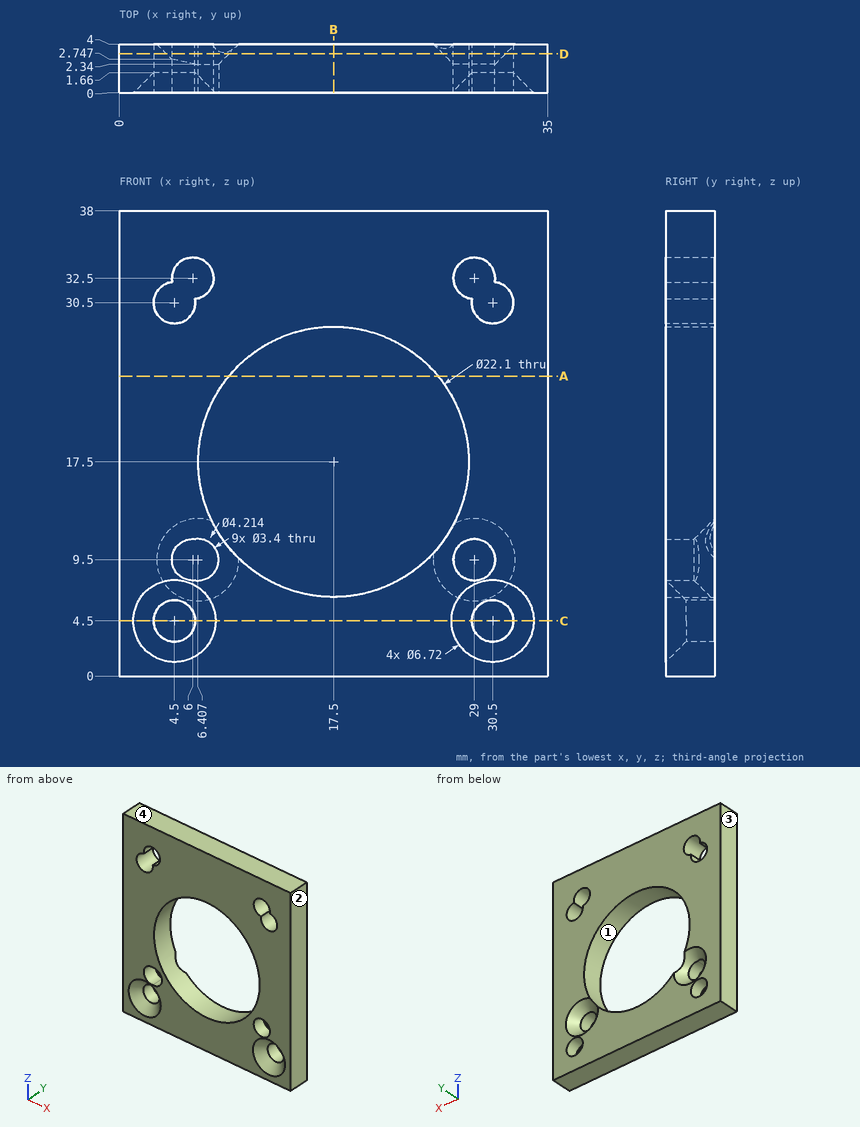
The drawing under review shows one solid part. Ordinate dimensions are in mm from its lowest x, y, z. Coordinates: 2 decimals unless noted, no trailing zeros. Order: outer loops, then holes, each group sorted by start corner. A loop starts at its lowest first (then second) coordinate and runs counter-clockwise, first axis right, second up. Notation, with made-up numbers: (-11.75, -26) -> (32.25, -26) arc R21 cw to (32.25, -13) -> close; hole circle Ø2 at (17, 13.25). An arc over 180 degrees is marked (long way). Answer in a Markdown table with one row per item. Add a question column.
Item 1: Clearance check with flat-ended pins moving along their axes: pin 1 (2 mm diameter, centred on x = 6, z = 32.5, fed in from +Y); pin 2 (5.5 mm diameter, centred on x = 4.5, z = 4.5, fed in from -Y); pin 3 (5.5 mm diameter, centred on x = 6.41, z = 9.5, fed in from +Y). State where each tip first meets the part, or that it passes through.
Item 2: To check wall thickness, follow probe 1 along X at (y, z) = (2.95, 30.5); probe 2 along X at (y, z) = (0.4, 32.5); probe 3 along Z at (x, y) = (30.5, 1.25). State the ranges of each line that lie inside material, in increasing order.
Item 3: Mouldability with a two-part tool opening along X and no side actions: class the marked faces 1, 2, 3 and 4 as +X half, -X half, draft (parallel to the pull), parting line (faces both ways), or undercut.
Item 4: We need section A-A on z = 24.5. Write out the cut boundary in (x, y).
Item 5: We need section C-C on z = 4.5. Write out the cut boundary in (x, y), plus the area to 3 significant figures.
Item 6: We need section D-D on y = 3.2. Write out the cut boundary in (x, z).
Item 7: We need section B-B on x = 17.5. Write out the cut boundary in (y, z), plus the area to 3 significant figures.
Final values:
| question | item | result |
|---|---|---|
| 1 | pin 1 | passes through |
| 1 | pin 2 | stops at y = 0.61 |
| 1 | pin 3 | stops at y = 3.39 |
| 2 | probe 1 | x = 0 to 2.8, 6.2 to 28.8, 32.2 to 35 |
| 2 | probe 2 | x = 0 to 4.3, 7.7 to 27.3, 30.7 to 35 |
| 2 | probe 3 | z = 0 to 2.39, 6.61 to 8.7, 10.3 to 28.8, 33.3 to 38 |
| 3 | face 1 | undercut |
| 3 | face 2 | +X half |
| 3 | face 3 | -X half |
| 3 | face 4 | draft |
| 4 | outline | (0, 0) -> (8.95, 0) -> (8.95, 4) -> (0, 4) -> close; (26.05, 0) -> (35, 0) -> (35, 4) -> (26.05, 4) -> close |
| 5 | outline | (0, 0) -> (1.14, 0) -> (2.8, 1.66) -> (2.8, 4) -> (0, 4) -> close; (6.2, 1.66) -> (7.86, 0) -> (27.14, 0) -> (28.8, 1.66) -> (28.8, 4) -> (6.2, 4) -> close; (32.2, 1.66) -> (33.86, 0) -> (35, 0) -> (35, 4) -> (32.2, 4) -> close |
| 5 | area | 107 mm2 |
| 6 | outline | (0, 0) -> (35, 0) -> (35, 38) -> (0, 38) -> close; hole circle Ø3.4 at (4.5, 4.5); hole circle Ø5.12 at (6.41, 9.5); hole (4.33, 32.19) arc R1.7 ccw (long way) to (6.17, 30.81) arc R1.7 ccw (long way) to start; hole circle Ø22.1 at (17.5, 17.5); hole circle Ø5.12 at (29, 9.5); hole circle Ø3.4 at (30.5, 4.5); hole (28.83, 30.81) arc R1.7 ccw (long way) to (30.67, 32.19) arc R1.7 ccw (long way) to start |
| 7 | outline | (0, 0) -> (4, 0) -> (4, 6.45) -> (0, 6.45) -> close; (0, 28.55) -> (4, 28.55) -> (4, 38) -> (0, 38) -> close |
| 7 | area | 63.6 mm2 |
